from build123d import *

# Parameters (mm, degrees)
BOSS_EXTRUDE1_DEPTH     = 3
SKETCH5_W               = 150
SKETCH5_H               = 20
BOSS_EXTRUDE2_DEPTH     = 3
MIRROR2_COPY_1_SKETCH_W = 150
MIRROR2_COPY_1_SKETCH_H = 20
MIRROR2_COPY_1_DEPTH    = 3
SKETCH6_W               = 23
SKETCH6_H               = 150
BOSS_EXTRUDE3_DEPTH     = 3
MIRROR4_COPY_1_SKETCH_W = 23
MIRROR4_COPY_1_SKETCH_H = 150
MIRROR4_COPY_1_DEPTH    = 3
MIRROR4_COPY_2_SKETCH_W = 23
MIRROR4_COPY_2_SKETCH_H = 150
MIRROR4_COPY_2_DEPTH    = 3
FILLET1_R               = 2
SKETCH4_W               = 35
SKETCH4_H               = 115
CUT_EXTRUDE1_DEPTH      = 10
TAP_DRILL_FOR_M3_TAP2_D = 2.5
TAP_DRILL_FOR_M3_TAP3_D = 2.5
M3_CLEARANCE_HOLE1_D    = 3.4
M8_CLEARANCE_HOLE1_D    = 9
CUT_EXTRUDE2_DEPTH      = 20
CUT_EXTRUDE2_DEPTH_BACK = 3


with BuildPart() as part:
    # Sketch1 → Boss-Extrude1 (new body)
    with BuildSketch(Plane.XY):
        Polygon((0, 195.984444731), (-138.581929877, 138.581929877), (-195.984444731, 0), (-138.581929877, -138.581929877), (0, -195.984444731), (138.581929877, -138.581929877), (195.984444731, 0), (138.581929877, 138.581929877), align=None)
    boss_extrude1 = extrude(amount=BOSS_EXTRUDE1_DEPTH)

    # Sketch5 → Boss-Extrude2 (add)
    with BuildSketch(Plane(origin=(-69.290964938, -167.283187304, 0), x_dir=(0.923879533, -0.382683432, 0), z_dir=(-0.382683432, -0.923879533, 0))):
        with Locations((0, -10)):
            Rectangle(SKETCH5_W, SKETCH5_H)
    boss_extrude2 = extrude(amount=-BOSS_EXTRUDE2_DEPTH)

    # Mirror1: Boss-Extrude2 across plane
    add(boss_extrude2.mirror(Plane.ZX))

    # Mirror2: Boss-Extrude2 across plane
    add(boss_extrude2.mirror(Plane(origin=(0, 0, 0), x_dir=(0, 0, 1), z_dir=(1, 0, 0))))

    # Mirror2 copy 1 sketch → Mirror2 copy 1 (add)
    with BuildSketch(Plane(origin=(69.290964938, 167.283187304, 0), x_dir=(-0.923879533, 0.382683432, 0), z_dir=(0.382683432, 0.923879533, 0))):
        with Locations((0, -10)):
            Rectangle(MIRROR2_COPY_1_SKETCH_W, MIRROR2_COPY_1_SKETCH_H)
    extrude(amount=-MIRROR2_COPY_1_DEPTH)

    # Sketch6 → Boss-Extrude3 (add)
    with BuildSketch(Plane(origin=(-167.283187304, -69.290964938, 0), x_dir=(0, 0, 1), z_dir=(-0.923879533, -0.382683432, 0))):
        with Locations((-8.5, 0)):
            Rectangle(SKETCH6_W, SKETCH6_H)
    boss_extrude3 = extrude(amount=-BOSS_EXTRUDE3_DEPTH)

    # Mirror3: Boss-Extrude3 across plane
    add(boss_extrude3.mirror(Plane.ZX))

    # Mirror4: Boss-Extrude1 across plane
    add(boss_extrude1.mirror(Plane(origin=(0, 0, 0), x_dir=(0, 0, 1), z_dir=(1, 0, 0))))

    # Mirror4 copy 1 sketch → Mirror4 copy 1 (add)
    with BuildSketch(Plane(origin=(167.283187304, 69.290964938, 0), x_dir=(0, 0, 1), z_dir=(0.923879533, 0.382683432, 0))):
        with Locations((-8.5, 0)):
            Rectangle(MIRROR4_COPY_1_SKETCH_W, MIRROR4_COPY_1_SKETCH_H)
    extrude(amount=-MIRROR4_COPY_1_DEPTH)

    # Mirror4 copy 2 sketch → Mirror4 copy 2 (add)
    with BuildSketch(Plane(origin=(167.283187304, -69.290964938, 0), x_dir=(0, 0, 1), z_dir=(0.923879533, -0.382683432, 0))):
        with Locations((-8.5, 0)):
            Rectangle(MIRROR4_COPY_2_SKETCH_W, MIRROR4_COPY_2_SKETCH_H)
    extrude(amount=-MIRROR4_COPY_2_DEPTH)

    # Fillet1
    fillet1_edges = [part.edges().sort_by_distance(p)[0] for p in [
        (-164.511548707, -68.142914641, 0),
        (-164.511548707, 68.142914641, 0),
        (164.511548707, 68.142914641, 0),
        (164.511548707, -68.142914641, 0),
        (-68.142914641, 164.511548707, 0),
        (68.142914641, 164.511548707, 0),
        (-68.142914641, -164.511548707, 0),
        (68.142914641, -164.511548707, 0),
    ]]
    fillet(fillet1_edges, radius=FILLET1_R)

    # Sketch4 → Cut-Extrude1 (cut)
    with BuildSketch(Plane(origin=(0, 0, 0), x_dir=(-1, 0, 0), z_dir=(0, 0, -1))):
        with Locations((-142.5, 0)):
            Rectangle(SKETCH4_W, SKETCH4_H)
        with Locations((125, 0)):
            Rectangle(SKETCH4_W, SKETCH4_H)
    extrude(amount=-CUT_EXTRUDE1_DEPTH, mode=Mode.SUBTRACT)

    # Tap Drill for M3 Tap2 (through all)
    with Locations(Plane(origin=(0, 0, 0), x_dir=(-1, 0, 0), z_dir=(0, 0, -1))):
        with Locations((-19.343368816, -169.062877249), (20.628515923, -169.078590597)):
            Hole(TAP_DRILL_FOR_M3_TAP2_D / 2)

    # Tap Drill for M3 Tap3 (through all)
    with Locations(Plane(origin=(0, 0, 0), x_dir=(-1, 0, 0), z_dir=(0, 0, -1))):
        with Locations((-20, -78.890298866), (20, -78.890298866)):
            Hole(TAP_DRILL_FOR_M3_TAP3_D / 2)

    # M3 Clearance Hole1 (through all)
    with Locations(Plane.XY.offset(3)):
        with Locations((-49.680592478, -98.01502722), (-71.876231555, -151.600040105), (-117.146328648, -132.848551919), (-94.950689571, -79.263539034)):
            Hole(M3_CLEARANCE_HOLE1_D / 2)

    # M8 Clearance Hole1 (through all)
    with Locations(Plane.XY.offset(3)):
        with Locations((111.402419859, -117.376896871), (-117.146328648, -132.848551919)):
            Hole(M8_CLEARANCE_HOLE1_D / 2)

    # Sketch21 → Cut-Extrude2 (cut, two sides)
    with BuildSketch(Plane(origin=(0, 0, 0), x_dir=(-1, 0, 0), z_dir=(0, 0, -1))) as cut_extrude2_sk:
        Polygon((0, -195.984444731), (-50.931031111, -174.8881209), (49.535442442, -175.466192654), align=None)
    extrude(amount=CUT_EXTRUDE2_DEPTH, mode=Mode.SUBTRACT)
    extrude(cut_extrude2_sk.sketch, amount=-CUT_EXTRUDE2_DEPTH_BACK, mode=Mode.SUBTRACT)


solid = part.part
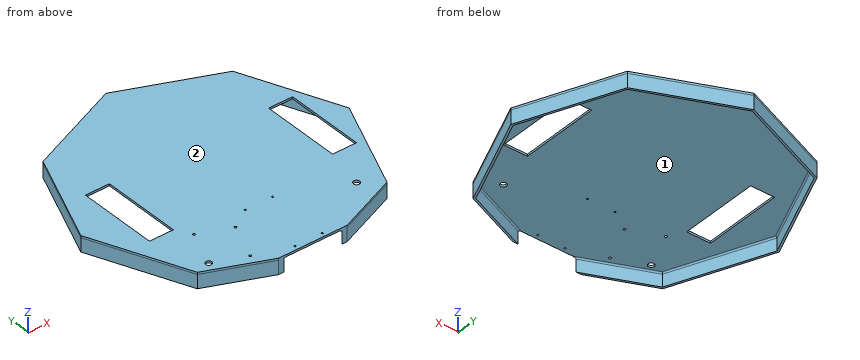
The listing builds one solid part. Answer for the finished solid, in the listing's coordinates (mm). Face numbers are marked on the shaded views. Round coordinates to 2 decimals unless told otherwise and drop trailing zeros. Write each loop counter-clockwise with the first axis right and the second up, starting at its lowest first coordinate (ties: lowest second). Pieces come first, ordered by that corner, then holes. Notation, with made-up numbers: (11, 1) - (20, 1) arc R19 cw to (20, 28) - close; hole circle Ø7 at (-39, 83.25). An arc over 180 degrees is marked (long way). Use a Markdown table: item, result. Add a question column.
1. The part is cut by section A-A (z = -11.5). Write down the section's boundary in (x, y).
2. The part is cut by section B-B (y = 13). Give the number of separate pieces and of enclosed holes in the cut face, and give its area (3 significant figures).
3. Flat-ended cylindrical pins translate along their axes: P1, Ø12, axis at x = -12, z = -2, coming from the +Y side; P2, Ø1.5, axis at y = 11.5, z = 1.5, coming from the +X side; P3, Ø3.5, axis at y = -13, z = 1, coming from the -X side. Find the tip coordinate at first contact, or state that the pin passes through.
4. For a pull along Y with two mould halves and no side action, classify the marked faces 1 and 2 as +Y half, -Y half, draft (parallel to the pull), parting line (faces both ways), or undercut.
5. Consider line 1 (X direction, y = 46.5, z = 1.75); line 2 (Y direction, x = 20, z = 1.05); line 3 (Z direction, x = 25, y = 115). Determine where each line is inside the solid, lowest interval first.
Reported:
| question | item | result |
|---|---|---|
| 1 | outline | (-195.98, 0) - (-138.58, -138.58) - (-49.54, -175.47) - (-41.8, -175.42) - (-136.29, -136.29) - (-192.74, 0) - (-136.29, 136.29) - (0, 192.74) - (136.29, 136.29) - (192.74, 0) - (136.29, -136.29) - (42.98, -174.93) - (50.93, -174.89) - (138.58, -138.58) - (195.98, 0) - (138.58, 138.58) - (0, 195.98) - (-138.58, 138.58) - close |
| 2 | separate pieces | 3 |
| 2 | enclosed holes | 0 |
| 2 | area | 1,070 mm^2 |
| 3 | P1 | y = 193.5 |
| 3 | P2 | x = 191.53 |
| 3 | P3 | x = -191.32 |
| 4 | face 1 | undercut |
| 4 | face 2 | draft |
| 5 | line 1 | -176.72 to -142.5, -107.5 to 125, 160 to 176.72 |
| 5 | line 2 | -175.07 to -170.13, -168 to -80.14, -77.64 to 187.7 |
| 5 | line 3 | 0 to 3 |
